Build history of the part. All positions in model axes, mm. Give positions to 0.01 mm unless a question says otherwise; leave off trailing zeros. Loops run counter-clockwise (first coordinate to the right, second up) from the corner with the lowest first, then second, coordinate; pieces in that order, holes last.
1) Band-saw the part on C-C on z = -3. List the corners of the cut face in (x, y) (1 decimal), then the cut area to 3 significant figures.
2) Flat gauge pins, fed straight in: P1, Ø7, axis at x = -76.5, z = -20.5, coming from the +Y side; P2, Ø1.5, axis at x = -100.5, z = 24.5, coming from the -Y side; P3, Ø1, axis at y = 6, z = -13.5, coming from the +X side; P4, Ø6, axis at x = -225, z = -20, coming from the +Y side. Where does each tip first touch, or does it go through?
3) Two-plate mould, pull along Y, no slides. Class faces 1 (the flat face through (-5, 0.914, 0)), 2 (the flat face through (5, 4.636, 1)): +Y half, -Y half, draft (parallel to the pull), parting line (faces both ways), or undercut.
4) Band-saw the part on A-A on y = 7. List the corners of the cut face in (x, z) (3 decimals), then the cut area to 3 significant figures.
5) Wall check: line 1 (Z direction, x = -75, y = 3.1); line 2 (Z direction, x = -17.5, y = 10); line 3 (Z direction, x = 375, y = 1.9). Give the ranges that are in metal, low to high.
```python
from build123d import *

# Parameters (mm, degrees)
SKETCH1_W           = 781.05
SKETCH1_H           = 80.1751
BOSS_EXTRUDE1_DEPTH = 10.922
SKETCH2_W           = 781.05
SKETCH2_H           = 9.0297
SKETCH2_H_2         = 24.4221
CUT_EXTRUDE1_DEPTH  = 0.9144
FILLET1_R           = 0.762
CUT_EXTRUDE2_DEPTH  = 783.154335313
SKETCH6_R           = 2.286
CUT_EXTRUDE4_DEPTH  = 393.627440931
LPATTERN1_COUNT     = 5
LPATTERN1_PITCH     = 150
LPATTERN2_COUNT     = 4
LPATTERN2_PITCH     = 150
SKETCH7_R           = 4.318
CUT_EXTRUDE5_DEPTH  = 2.159
LPATTERN3_COUNT     = 6
LPATTERN3_PITCH     = 150


with BuildPart() as part:
    # Sketch1 → Boss-Extrude1 (new body)
    with BuildSketch(Plane(origin=(0, 0, 0), x_dir=(1, 0, 0), z_dir=(0, 1, 0))):
        Rectangle(SKETCH1_W, SKETCH1_H)
    extrude(amount=BOSS_EXTRUDE1_DEPTH)

    # Sketch2 → Cut-Extrude1 (cut)
    with BuildSketch(Plane.XZ):
        with Locations((0, 32.4612)):
            Rectangle(SKETCH2_W, SKETCH2_H)
        Rectangle(SKETCH2_W, SKETCH2_H_2)
        with Locations((0, -32.4612)):
            Rectangle(SKETCH2_W, SKETCH2_H)
    extrude(amount=-CUT_EXTRUDE1_DEPTH, mode=Mode.SUBTRACT)

    # Fillet1
    fillet1_edges = [part.edges().sort_by_distance(p)[0] for p in [
        (0, 0.9144, 27.94635),
        (0, 0.9144, 36.97605),
        (0, 0.9144, -12.21105),
        (0, 0.9144, 12.21105),
        (0, 0.9144, -36.97605),
        (0, 0.9144, -27.94635),
    ]]
    fillet(fillet1_edges, radius=FILLET1_R)

    # Sketch3 → Cut-Extrude2 (cut, through all)
    with BuildSketch(Plane(origin=(390.525, 0, 0), x_dir=(0, 0, -1), z_dir=(1, 0, 0))):
        Polygon((-29.92755, 10.922), (-29.92755, 8.89), (-37.67455, 8.89), (-37.67455, 4.6355), (37.67455, 4.6355), (37.67455, 8.89), (29.92755, 8.89), (29.92755, 10.922), align=None)
    extrude(amount=-CUT_EXTRUDE2_DEPTH, mode=Mode.SUBTRACT)

    # Sketch6 → Cut-Extrude4 (cut, through all)
    with BuildSketch(Plane(origin=(0, 4.6355, 0), x_dir=(1, 0, 0), z_dir=(0, 1, 0))):
        with Locations(Location((75, -20, 0), (0, 0, 270))):
            Circle(SKETCH6_R)
        with Locations(Location((75, 20, 0), (0, 0, 270))):
            Circle(SKETCH6_R)
    cut_extrude4 = extrude(amount=-CUT_EXTRUDE4_DEPTH, mode=Mode.SUBTRACT)

    # LPattern1: Cut-Extrude4 ×5
    with Locations(*[(i * LPATTERN1_PITCH, 0, 0) for i in range(1, LPATTERN1_COUNT)]):
        add(cut_extrude4, mode=Mode.SUBTRACT)

    # LPattern2: Cut-Extrude4 ×4
    with Locations(*[(-i * LPATTERN2_PITCH, 0, 0) for i in range(1, LPATTERN2_COUNT)]):
        add(cut_extrude4, mode=Mode.SUBTRACT)

    # Sketch7 → Cut-Extrude5 (cut)
    with BuildSketch(Plane(origin=(0, 4.6355, 0), x_dir=(1, 0, 0), z_dir=(0, 1, 0))):
        with Locations(Location((375, -20, 0), (0, 0, 270))):
            Circle(SKETCH7_R)
        with Locations(Location((375, 20, 0), (0, 0, 270))):
            Circle(SKETCH7_R)
    cut_extrude5 = extrude(amount=-CUT_EXTRUDE5_DEPTH, mode=Mode.SUBTRACT)

    # LPattern3: Cut-Extrude5 ×6
    with Locations(*[(-i * LPATTERN3_PITCH, 0, 0) for i in range(1, LPATTERN3_COUNT)]):
        add(cut_extrude5, mode=Mode.SUBTRACT)


solid = part.part
```
Findings below:
1. outline: (-390.5, 0.9) - (390.5, 0.9) - (390.5, 4.6) - (-390.5, 4.6) - close
1. area: 2,910 mm2
2. P1: stops at y = 4.64
2. P2: stops at y = 0
2. P3: passes through
2. P4: stops at y = 2.48
3. face 1: -Y half
3. face 2: undercut
4. outline: (-390.525, -40.088) - (390.525, -40.088) - (390.525, -37.675) - (-390.525, -37.675) - close; (-390.525, 37.675) - (390.525, 37.675) - (390.525, 40.088) - (-390.525, 40.088) - close
4. area: 3,770 mm2
5. line 1: z = -40.09 to -24.32, -15.68 to 15.68, 24.32 to 40.09
5. line 2: z = -40.09 to -29.93, 29.93 to 40.09
5. line 3: z = -40.09 to -22.29, -17.71 to 17.71, 22.29 to 40.09
